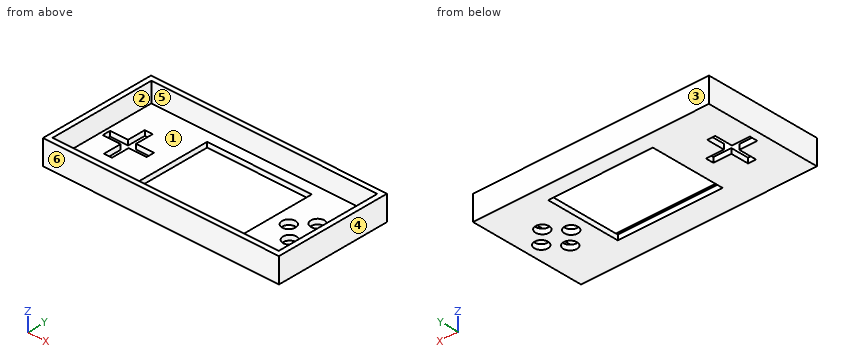
from build123d import *

# Parameters (mm, degrees)
F0_W     = 115.0112
F0_H     = 54.0004
F1_DEPTH = 10
F2_T     = 2.54
F3_W     = 53.34
F3_H     = 38.1
F4_DEPTH = 12.7
F6_DEPTH = 12.7
F7_R     = 3.429
F8_DEPTH = 12.7


with BuildPart() as f1:
    # F0 (on Top) → F1 (new body)
    with BuildSketch(Plane.XY):
        with Locations((1.2398222461, -0.5762684962)):
            Rectangle(F0_W, F0_H)
    extrude(amount=F1_DEPTH)

    # F2
    f2_openings = [f1.faces().sort_by_distance(p)[0] for p in [
        (1.239822, -0.576268, 10),
    ]]
    offset(amount=F2_T, openings=f2_openings, kind=Kind.INTERSECTION)

    # F3 (on face) → F4 (cut, symmetric)
    with BuildSketch(Plane(origin=(0, 0, -2.54), x_dir=(1, 0, 0), z_dir=(0, 0, -1))):
        with Locations((3.7798222461, -1.9637315038)):
            Rectangle(F3_W, F3_H)
    extrude(amount=F4_DEPTH, both=True, mode=Mode.SUBTRACT)

    # F5 (on Top) → F6 (cut, symmetric)
    with BuildSketch(Plane.XY):
        Polygon((-45.4199777539, -2.032), (-45.4199777539, -11.176), (-41.3559777539, -11.176), (-41.3559777539, -2.032), (-32.2119777539, -2.032), (-32.2119777539, 2.032), (-41.3559777539, 2.032), (-41.3559777539, 11.176), (-45.4199777539, 11.176), (-45.4199777539, 2.032), (-54.5639777539, 2.032), (-54.5639777539, -2.032), align=None)
    extrude(amount=F6_DEPTH, both=True, mode=Mode.SUBTRACT)

    # F7 (on Top) → F8 (cut, symmetric)
    with BuildSketch(Plane.XY):
        with Locations((45.8676222461, -7.62)):
            Circle(F7_R)
        with Locations((53.4876222461, 0)):
            Circle(F7_R)
        with Locations((45.8676222461, 7.62)):
            Circle(F7_R)
        with Locations((38.2476222461, 0)):
            Circle(F7_R)
    extrude(amount=F8_DEPTH, both=True, mode=Mode.SUBTRACT)


solid = f1.part
Source: CAD feature listing. Evaluate the final solid. Frame: model axes, mm. Face numbers are marked on the shaded views. A direction names the side the tool comes from. Round coordinates to 2 decimals unless told otherwise and drop trailing zeros. Loops run counter-clockwise (first coordinate to the right, second up) from the corner with the lowest first, then second, coordinate; pieces in that order, holes last. Notation, with made-up numbers: M 66.5,77 L 101.5,77 A33 ccw 101.5,105 Z; hole C 44,54 d10. An arc over 180 degrees is marked long. Answer as CSV lines item,"result".
Q1. Pull-direction query (X, two-part tool) for the marked faces 1, 2, 3 and 4; classes: +X half, -X half, draft (parallel to the pull), parting line (faces both ways), or undercut.
Verdict:
face 1,"undercut"
face 2,"undercut"
face 3,"draft"
face 4,"+X half"
Q2. Line query: line 1 along Y through (x, z) = (-41, 3.25); line 2 along X through (y, z) = (22.5, 4.25); line 3 along X through (y, z) = (-3, -1.5). Output: solid intervals per line, ascending.
Verdict:
line 1,"y = -30.12 to -27.58, 26.42 to 28.96"
line 2,"x = -58.81 to -56.27, 58.75 to 61.29"
line 3,"x = -58.81 to -45.42, -41.36 to -22.89, 30.45 to 36.59, 39.91 to 51.83, 55.15 to 61.29"
Q3. Cut plane D-D (z = 7.25). Return the cut outline in (x, y).
Verdict:
outline,"M -58.81,-30.12 L 61.29,-30.12 L 61.29,28.96 L -58.81,28.96 Z; hole M -56.27,-27.58 L 58.75,-27.58 L 58.75,26.42 L -56.27,26.42 Z"
Q4. Cut plane C-C (y = 0). Return the cut outline in (x, z).
Verdict:
outline,"M -58.81,-2.54 L -54.56,-2.54 L -54.56,0 L -56.27,0 L -56.27,10 L -58.81,10 Z; M -32.21,-2.54 L -22.89,-2.54 L -22.89,0 L -32.21,0 Z; M 30.45,-2.54 L 34.82,-2.54 L 34.82,0 L 30.45,0 Z; M 41.68,-2.54 L 50.06,-2.54 L 50.06,0 L 41.68,0 Z; M 56.92,-2.54 L 61.29,-2.54 L 61.29,10 L 58.75,10 L 58.75,0 L 56.92,0 Z"
Q5. Cut plane B-B (x = 26.5). Return the cut outline in (y, z), plus the area to 3 significant figures.
Verdict:
outline,"M -30.12,-2.54 L -17.09,-2.54 L -17.09,0 L -27.58,0 L -27.58,10 L -30.12,10 Z; M 21.01,-2.54 L 28.96,-2.54 L 28.96,10 L 26.42,10 L 26.42,0 L 21.01,0 Z"
area,"104 mm^2"
Q6. Reachability of the marked faces 5 and 6 from +Z, -Z, +X, -X, +Y, -Y: full face, straight path, thin tool, end or side. Return the list, or none.
Verdict:
face 5,"+Z"
face 6,"+Z, -Z, +X, -X, -Y"
Q7. Contact query for a flat-ended pin moving along its axis: pin 1 (6 mm diameter, centred on x = -41.5, y = -24, fed in from +Z). Output: stop coordinate, or through.
Verdict:
pin 1,"stops at z = 0"
Q8. Cut plane A-A (y = 7.62). Return the cut outline in (x, z).
Verdict:
outline,"M -58.81,-2.54 L -45.42,-2.54 L -45.42,0 L -56.27,0 L -56.27,10 L -58.81,10 Z; M -41.36,-2.54 L -22.89,-2.54 L -22.89,0 L -41.36,0 Z; M 30.45,-2.54 L 42.44,-2.54 L 42.44,0 L 30.45,0 Z; M 49.3,-2.54 L 61.29,-2.54 L 61.29,10 L 58.75,10 L 58.75,0 L 49.3,0 Z"
